from build123d import *

# Parameters (mm, degrees)
SKETCH1_W           = 24.5
SKETCH1_H           = 25
BOSS_EXTRUDE1_DEPTH = 1
SKETCH2_W           = 6
SKETCH2_H           = 22
BOSS_EXTRUDE2_DEPTH = 3
SKETCH3_R           = 1
CUT_EXTRUDE1_DEPTH  = 18.757040857
SKETCH4_R           = 2
SKETCH4_W           = 13
SKETCH4_H           = 13
BOSS_EXTRUDE3_DEPTH = 4
SKETCH5_R           = 7
BOSS_EXTRUDE4_DEPTH = 12


with BuildPart() as part:
    # Sketch1 → Boss-Extrude1 (new body)
    with BuildSketch(Plane.XY):
        Rectangle(SKETCH1_W, SKETCH1_H)
    extrude(amount=BOSS_EXTRUDE1_DEPTH)

    # Sketch2 → Boss-Extrude2 (add)
    with BuildSketch(Plane.XY.offset(1)):
        with Locations((-9.25, 0)):
            Rectangle(SKETCH2_W, SKETCH2_H)
    extrude(amount=BOSS_EXTRUDE2_DEPTH)

    # Sketch3 → Cut-Extrude1 (cut, through all)
    with BuildSketch(Plane.XY.offset(1)):
        with Locations((10.25, 10.5)):
            Circle(SKETCH3_R)
        with Locations((10.25, -10.5)):
            Circle(SKETCH3_R)
        with Locations((-3.25, 10.5)):
            Circle(SKETCH3_R)
        with Locations((-3.25, -10.5)):
            Circle(SKETCH3_R)
    extrude(amount=-CUT_EXTRUDE1_DEPTH, mode=Mode.SUBTRACT)

    # Sketch4 → Boss-Extrude3 (add)
    with BuildSketch(Plane.XY.offset(1)):
        with Locations((3.25, 9.5)):
            Circle(SKETCH4_R)
        with BuildLine():
            Line((5.25, 6.5), (5.25, 9.5))
            ThreePointArc((5.25, 9.5), (3.25, 7.5), (1.25, 9.5))
            Line((1.25, 9.5), (1.25, 6.5))
            Line((1.25, 6.5), (5.25, 6.5))
        make_face()
        with Locations((3.25, 0)):
            Rectangle(SKETCH4_W, SKETCH4_H)
        with Locations((3.25, -9.5)):
            Circle(SKETCH4_R)
        with BuildLine():
            Line((5.25, -9.5), (5.25, -6.5))
            Line((5.25, -6.5), (1.25, -6.5))
            Line((1.25, -6.5), (1.25, -9.5))
            ThreePointArc((1.25, -9.5), (3.25, -7.5), (5.25, -9.5))
        make_face()
    extrude(amount=BOSS_EXTRUDE3_DEPTH)

    # Sketch5 → Boss-Extrude4 (add)
    with BuildSketch(Plane.XY.offset(5)):
        with Locations(Location((3.25, 0, 0), (0, 0, 158.213210702))):
            Circle(SKETCH5_R)
    extrude(amount=BOSS_EXTRUDE4_DEPTH)

    # Sketch7 → Revolve1 (revolve)
    with BuildSketch(Plane(origin=(0, 0, 0), x_dir=(1, 0, 0), z_dir=(0, 1, 0))):
        with BuildLine():
            Line((3.25, -17), (3.25, -20))
            add(Edge.make_bspline(
                [(-3.75, -17), (-1.521062197, -20.264896089), (3.25, -20)],
                knots=[0, 0, 0, 1, 1, 1], degree=2))
            Line((-3.75, -17), (3.25, -17))
        make_face()
    revolve(axis=Axis((3.25, 0, 17), (0, 0, 1)))


solid = part.part
Design review of the part built by this model. Coordinates are the model's own, in mm. A direction names the side the tool comes from. Give positions to 0.01 mm unless a question says otherwise; leave off trailing zeros. Write each loop counter-clockwise with the first axis right and the second up, starting at its lowest first coordinate (ties: lowest second). Pieces come first, ordered by that corner, then holes. Notation, with made-up numbers: M 37,60 L 85,60 A23 ccw 85,97 Z; hole C 57.25,-37 d5. An arc over 180 degrees is marked long. Return JSON: item names as keys, results as strings. Group by question number.
Item 1: Take a section at A-A (x = -7). Give the boundary of the cut face in (y, z), plus the area to 3 significant figures.
Item 2: The part is to be moulded in two halves that separate along Y. For faces 6 (the flat face through (-0.2, -12.5, 0.5)), 7 (the cylindrical face through (-3.38, -9.51, 0.51)), 8 (the cylindrical face through (-3.987, 11.176, 0.507)), 9 (the flat face through (1.25, 8, 3)), say which applies: pulls with the +Y half, pulls with the -Y half, needs draft (parallel to the pull), parting line crosses it, or undercut.
Item 3: Tool access review of faces 1 (the cylindrical face through (3.3, 11.5, 3)), 2 (the flat face through (-9, -11, 2)), 3 (the flat face through (-3.25, 0, 3)), 4 (the flat face through (-9, 11, 2)), 5 (the cylindrical face through (7.2, 5.78, 10.92)): name each direction out of +Z, -Z, +X, -X, +Y, -Y from which nothing blocks a thin tool from reaching the whole face with its end or side.
Item 4: Clearance check with flat-ended pins moving along their axes: pin 1 Ø0.9 at (x, z) = (-10, 2.5) entering from +Y; pin 2 Ø4 at (x, y) = (1, -5) entering from +Z; pin 3 Ø5 at (x, y) = (5, 8) entering from -Z; pin 4 Ø3 at (y, z) = (4, 9.5) entering from +X. State where each tip first meets the part, or that it passes through.
Item 5: Wall thickness on line 1 along Y through (x, z) = (10.25, 0.55); line 2 along Z through (x, y) = (-8.5, 5.75); line 3 along Z through (x, y) = (-6, -8): over which ranges is each line inside the solid? List them lowest first.
Item 6: Take a section at B-B (y = -10.5). Give the boundary of the cut face in (x, z), plus the area to 3 significant figures.
Item 7: Take a section at C-C (z = 10.75). Give the boundary of the cut face in (x, y).
Return value:
{
 "1": {"outline": "M -12.5,0 L 12.5,0 L 12.5,1 L 11,1 L 11,4 L -11,4 L -11,1 L -12.5,1 Z", "area": "91.0 mm2"},
 "2": {"face 6": "pulls with the -Y half", "face 7": "undercut", "face 8": "undercut", "face 9": "needs draft"},
 "3": {"face 1": "+Z, +Y", "face 2": "+Z, -X, -Y", "face 3": "+Y, -Y", "face 4": "+Z, -X, +Y", "face 5": "+Z"},
 "4": {"pin 1": "stops at y = 11", "pin 2": "stops at z = 19.62", "pin 3": "stops at z = 0", "pin 4": "stops at x = 9.79"},
 "5": {"line 1": "y = -12.5 to -11.5, -9.5 to 9.5, 11.5 to 12.5", "line 2": "z = 0 to 4", "line 3": "z = 0 to 1"},
 "6": {"outline": "M -12.25,0 L -4.25,0 L -4.25,1 L -6.25,1 L -6.25,4 L -12.25,4 Z; M -2.25,0 L 9.25,0 L 9.25,1 L 4.98,1 L 4.98,5 L 1.52,5 L 1.52,1 L -2.25,1 Z; M 11.25,0 L 12.25,0 L 12.25,1 L 11.25,1 Z", "area": "52.4 mm2"},
 "7": {"outline": "C 3.25,0 d14"}
}
